from build123d import *

# Parameters (mm, degrees)
SKETCH1_R                    = 46.99
BOSS_EXTRUDE1_DEPTH          = 330.2
SKETCH2_W                    = 44.45
SKETCH2_H                    = 44.45
CUT_EXTRUDE1_DEPTH           = 330.2
CUT_EXTRUDE1_DRAFT           = -2.5
CUT_EXTRUDE2_START           = -330.2
SKETCH3_R                    = 1.905
CUT_EXTRUDE2_DEPTH           = 330.2
CUT_EXTRUDE4_START           = -165.1
CUT_EXTRUDE4_DEPTH           = 165.1
SKETCH8_R                    = 4.8895
CUT_EXTRUDE5_DEPTH           = 4.7879
CUT_EXTRUDE5_DRAFT           = -45
CUT_EXTRUDE5_PROFILE_2_DEPTH = 4.7879
CUT_EXTRUDE5_PROFILE_2_DRAFT = -45


with BuildPart() as part:
    # Sketch1 → Boss-Extrude1 (new body)
    with BuildSketch(Plane(origin=(0, 0, 0), x_dir=(1, 0, 0), z_dir=(0, 1, 0))):
        with Locations(Location((0, 0, 0), (0, 0, 270))):
            Circle(SKETCH1_R)
    extrude(amount=BOSS_EXTRUDE1_DEPTH)


with BuildPart() as cut_extrude1_tool:
    # Sketch2 → Cut-Extrude1 (with draft: the straight prism first)
    with BuildSketch(Plane(origin=(0, 330.2, 0), x_dir=(1, 0, 0), z_dir=(0, 1, 0))):
        Rectangle(SKETCH2_W, SKETCH2_H)
    extrude(amount=-CUT_EXTRUDE1_DEPTH)
    # Cut-Extrude1: the draft: its side faces are tilted about the plane it starts from
    cut_extrude1_sides = [cut_extrude1_tool.faces().sort_by_distance(p)[0] for p in [
        (-22.225, 165.1, 0),
        (0, 165.1, 22.225),
        (22.225, 165.1, 0),
        (0, 165.1, -22.225),
    ]]
    draft(cut_extrude1_sides, Plane(origin=(0, 330.2, 0), x_dir=(1, 0, 0), z_dir=(0, 1, 0)), CUT_EXTRUDE1_DRAFT)


with BuildPart() as part_1:
    add(part.part)

    # Cut-Extrude1: cut by cut_extrude1_tool
    add(cut_extrude1_tool.part, mode=Mode.SUBTRACT)

    # Sketch3 → Cut-Extrude2 (cut)
    with BuildSketch(Plane(origin=(0, 330.2, 0), x_dir=(1, 0, 0), z_dir=(0, 1, 0)).offset(CUT_EXTRUDE2_START)):
        with Locations(Location((-26.9875, 26.9875, 0), (0, 0, 270))):
            Circle(SKETCH3_R)
        with BuildLine():
            Line((0, 12.7), (0, 46.99))
            ThreePointArc((0, 46.99), (33.226947648, -33.226947648), (-46.99, 0))
            Line((-46.99, 0), (-12.7, 0))
            Line((-12.7, 0), (0, 0))
            Line((0, 0), (0, 12.7))
        make_face()
    extrude(amount=CUT_EXTRUDE2_DEPTH, mode=Mode.SUBTRACT)

    # Sketch7 → Cut-Extrude4 (cut)
    with BuildSketch(Plane(origin=(0, 330.2, 0), x_dir=(1, 0, 0), z_dir=(0, 1, 0)).offset(CUT_EXTRUDE4_START)):
        with BuildLine():
            Line((0, 46.99), (0, 0))
            Line((0, 0), (-46.99, 0))
            ThreePointArc((-46.99, 0), (-33.226947648, 33.226947648), (0, 46.99))
        make_face()
    extrude(amount=CUT_EXTRUDE4_DEPTH, mode=Mode.SUBTRACT)


with BuildPart() as cut_extrude5_tool:
    # Sketch8 → Cut-Extrude5 (with draft: the straight prism first)
    with BuildSketch(Plane(origin=(0, 165.1, 0), x_dir=(1, 0, 0), z_dir=(0, 1, 0))):
        with Locations((-12.573, 30.48)):
            Circle(SKETCH8_R)
    extrude(amount=-CUT_EXTRUDE5_DEPTH)
    # Cut-Extrude5: the draft: its side faces are tilted about the plane it starts from
    cut_extrude5_sides = [cut_extrude5_tool.faces().sort_by_distance(p)[0] for p in [
        (-17.4625, 162.70605, -30.48),
    ]]
    draft(cut_extrude5_sides, Plane(origin=(0, 165.1, 0), x_dir=(1, 0, 0), z_dir=(0, 1, 0)), CUT_EXTRUDE5_DRAFT)


with BuildPart() as part_2:
    add(part_1.part)

    # Cut-Extrude5: cut by cut_extrude5_tool
    add(cut_extrude5_tool.part, mode=Mode.SUBTRACT)


with BuildPart() as cut_extrude5_profile_2_tool:
    # Sketch8 → Cut-Extrude5 profile 2 (with draft: the straight prism first)
    with BuildSketch(Plane(origin=(0, 165.1, 0), x_dir=(1, 0, 0), z_dir=(0, 1, 0))):
        with Locations((-30.48, 12.573)):
            Circle(SKETCH8_R)
    extrude(amount=-CUT_EXTRUDE5_PROFILE_2_DEPTH)
    # Cut-Extrude5 profile 2: the draft: its side faces are tilted about the plane it starts from
    cut_extrude5_profile_2_sides = [cut_extrude5_profile_2_tool.faces().sort_by_distance(p)[0] for p in [
        (-35.3695, 162.70605, -12.573),
    ]]
    draft(cut_extrude5_profile_2_sides, Plane(origin=(0, 165.1, 0), x_dir=(1, 0, 0), z_dir=(0, 1, 0)), CUT_EXTRUDE5_PROFILE_2_DRAFT)


with BuildPart() as part_3:
    add(part_2.part)

    # Cut-Extrude5 profile 2: cut by cut_extrude5_profile_2_tool
    add(cut_extrude5_profile_2_tool.part, mode=Mode.SUBTRACT)


solid = part_3.part
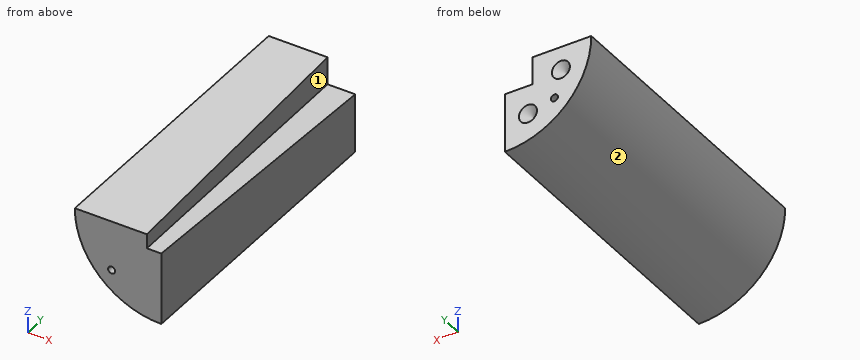
Read the model definition and answer for the solid it produces. Units are mm, in the model's axes. Face numbers are marked on the shaded views. A direction names the side the tool comes from. Round coordinates to 2 decimals unless told otherwise and drop trailing zeros. Loops run counter-clockwise (first coordinate to the right, second up) from the corner with the lowest first, then second, coordinate; pieces in that order, holes last. Notation, with made-up numbers: (44, -10.5) - (59, -10.5) arc R9 cw to (59, 0.5) - close; hole circle Ø9 at (-30.5, -23). An arc over 180 degrees is marked (long way). One line per question, with ' | ' between items. Start each with the question number.
Q1. Find the intervals of material crossed by L1, parallel to Z at x = -26, y = 58; L2, parallel to Z at x = -27, y = 123; L3, parallel to Z at x = -4.5, y = 103, in increasing order.
Q2. Section D-D on z = -43 is taken. Give the vertices of the cut face in (x, y).
Q3. For the marked faces 1 and 2, determine the directions among +Z, -Z, +X, -X, +Y, -Y from which every point of the face is accessible in a straight line to the end or side of a thin tool.
Q4. Section A-A on y = 150.5 is taken. Give the vertices of the cut face in (x, z) (1 decimal), plus the area to 3 significant figures.
Q5. Flat-ended cylindrical pins translate along their axes: pin 1 (5 mm diameter, centred on y = 23, z = -8.5, fed in from -X); pin 2 (5 mm diameter, centred on y = 23, z = -38, fed in from -X); pin 3 (8 mm diameter, centred on y = 18.5, z = -25, fed in from -X); pin 4 (6 mm diameter, centred on x = -33.5, z = -32, fed in from -Y). Find the tip coordinate at first contact, or state that the pin passes through.
Q6. Section C-C on y = 111 is taken. Give the vertices of the cut face in (x, z) (1 decimal), plus the area to 3 significant figures.
Q7. Section B-B on x = -41 is taken. Give the vertices of the cut face in (y, z), plus the area to 3 significant figures.
Established:
1) L1: -39.14 to -28.62, -25.36 to 0 | L2: -38.46 to -28.89, -25.08 to 0 | L3: -46.77 to -12.31
2) outline: (-18.95, 0) - (0, 0) - (0, 165.1) - (-18.95, 165.1) - close
3) face 1: +Z, +X, +Y | face 2: -Z, -X, +Y, -Y
4) outline: (-47, 0) arc R47 ccw to (0, -47) - (0, -14.4) - (-14.4, -14.4) - (-14.4, 0) - close; hole circle Ø3.8 at (-27, -27) | area: 1,520 mm²
5) pin 1: x = -46.61 | pin 2: x = -30.79 | pin 3: x = -42.04 | pin 4: y = 0
6) outline: (-47, 0) arc R47 ccw to (0, -47) - (0, -12.7) - (-12.7, -12.7) - (-12.7, 0) - close; hole circle Ø3.8 at (-27, -27) | area: 1,560 mm²
7) outline: (0, -22.96) - (165.1, -22.96) - (165.1, 0) - (0, 0) - close | area: 3,790 mm²
